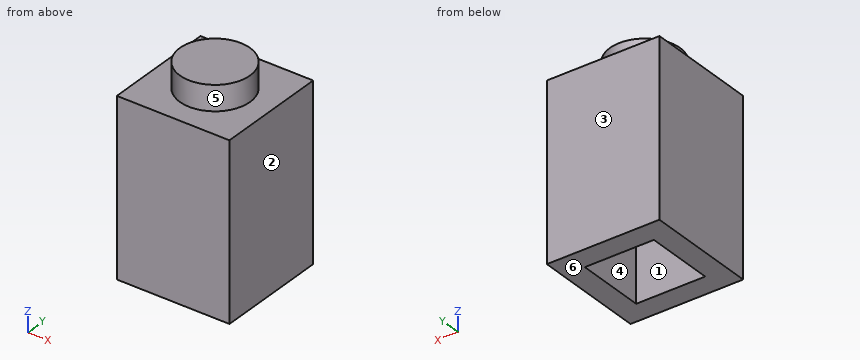
from build123d import *

# Parameters (mm, degrees)
F0_W     = 7.874
F0_H     = 7.874
F1_DEPTH = 12.1666
F2_T     = -1.524
F4_D     = 1.905
F4_DEPTH = 0.254
F4_TIP   = 0.5723197396
F5_R     = 2.4511
F6_DEPTH = 1.7526


with BuildPart() as f1:
    # F0 (on Top) → F1 (new body)
    with BuildSketch(Plane.XY):
        Rectangle(F0_W, F0_H)
    extrude(amount=F1_DEPTH)

    # F2
    f2_openings = [f1.faces().sort_by_distance(p)[0] for p in [
        (0, 0, 0),
    ]]
    offset(amount=F2_T, openings=f2_openings)

    # F4
    with Locations(Plane(origin=(0, 0, 10.6426), x_dir=(1, 0, 0), z_dir=(0, 0, -1))):
        with Locations((0, 0)):
            Hole(F4_D / 2, depth=F4_DEPTH)
            with Locations((0, 0, -(F4_DEPTH + F4_TIP / 2))):  # 118° drill point
                Cone(0, F4_D / 2, F4_TIP, mode=Mode.SUBTRACT)

    # F5 (on face) → F6 (join)
    with BuildSketch(Plane.XY.offset(12.1666)):
        Circle(F5_R)
    extrude(amount=F6_DEPTH)


solid = f1.part
Could you check a few things on this model? Use its own coordinates, in mm. Face numbers are marked on the shaded views. A direction names the side the tool comes from. Round coordinates to 2 decimals unless told otherwise and drop trailing zeros. Order: outer loops, then holes, each group sorted by start corner. A loop starts at its lowest first (then second) coordinate and runs counter-clockwise, first axis right, second up. Notation, with made-up numbers: M 61.25,49.5 L 102.25,49.5 A19 ccw 102.25,71.5 Z; hole C 41.25,41 d10. An arc over 180 degrees is marked long. One line per item, written item: value.
(1) If we mould it in two halves opening along Y, with no side actions, what happens to the marked faces 1, 2, 3 and 4? For each: released by +Y, released by -Y, zero draft, split by the parting line, or undercut.
Ans:
face 1: undercut
face 2: zero draft
face 3: released by +Y
face 4: undercut
(2) Imagine slicing it at D-D (z = 12.75). Write out the boundary of the cut face in (x, y).
Ans:
outline: C 0,0 d4.9
(3) I'm going to push a flat-ended pin straight in: P1, Ø1.1, axis at x = 0, y = 0, coming from the -Z side. Where does the tip first touch, or does it pass through?
Ans:
P1: stops at z = 11.14
(4) Imagine slicing it at B-B (y = 2). Write out the boundary of the cut face in (x, z), and give its area (3 significant figures).
Ans:
outline: M -3.94,0 L -2.41,0 L -2.41,10.64 L 2.41,10.64 L 2.41,0 L 3.94,0 L 3.94,12.17 L 1.42,12.17 L 1.42,13.92 L -1.42,13.92 L -1.42,12.17 L -3.94,12.17 Z
area: 49.4 mm^2
(5) Imagine slicing it at C-C (x = -2.75). Write out the boundary of the cut face in (y, z).
Ans:
outline: M -3.94,0 L 3.94,0 L 3.94,12.17 L -3.94,12.17 Z
(6) Which directions (+Z, -Z, +X, -X, +Y, -Y) give clear straight access to the entire face, cutting with the end or side of a thin tool? Please do the marked faces 5 and 6.
Ans:
face 5: +Z
face 6: -Z, +X, -X, +Y, -Y
(7) I need wall thicknesses on line 1 along Y through (x, z) = (-2.25, 5.75); line 2 along Z through (x, y) = (3.5, 2.75). Which ranges of each line are inside material? Lowest first, please. Write a range as from..to.
Ans:
line 1: y = -3.94..-2.41, 2.41..3.94
line 2: z = 0..12.17
(8) Imagine slicing it at A-A (z = 9.5). Write out the boundary of the cut face in (x, y).
Ans:
outline: M -3.94,-3.94 L 3.94,-3.94 L 3.94,3.94 L -3.94,3.94 Z; hole M -2.41,-2.41 L 2.41,-2.41 L 2.41,2.41 L -2.41,2.41 Z
